Autodesk Inventor part; units mm, degrees
ref_plane "YZ Plane" through (0, 0, 0) normal (1, 0, 0) x (0, 1, 0)
ref_plane "XZ Plane" through (0, 0, 0) normal (0, 1, 0) x (-1, 0, 0)
ref_plane "XY Plane" through (0, 0, 0) normal (0, 0, 1) x (1, 0, 0)
sketch "Sketch2" plane through (0, 0, 0) normal (1, 0, 0) x (0, 1, 0)
  line L0 (0, 0) -> (2.5, 0)
  line L1 (2.5, 0) -> (2.5, -5.3)
  line L2 (2.5, -5.3) -> (2.15, -5.3)
  line L3 (2.15, -5.3) -> (2.15, -14.7)
  line L4 (2.15, -14.7) -> (2.5, -14.7)
  line L5 (2.5, -14.7) -> (2.5, -20)
  line L6 (2.5, -20) -> (0, -20)
  line L7 (0, -20) -> (0, 0)
  dimension "d1" = 2.5
  dimension "d2" = 5.3
  dimension "d3" = 0.35
  dimension "d4" = 9.4
  dimension "d5" = 0.35
  dimension "d6" = 5.3
  dimension "d7" = 2.5
revolve "Revolution1" add sketch "Sketch2" angle 360 about axis through (0, 0, -20) along (0, 0, 1)
fillet "Fillet4" radius 0.4 2 edges at (0, -2.5, -20) (0, -2.5, 0)
fillet "Fillet5" radius 0.35 2 edges at (0, -2.5, -14.7) (0, -2.5, -5.3)
equation "\"d5\" = d3"
equation "\"d6\" = d2"
equation "\"d7\" = d1"
properties part number "Fusible de 2A"
Verification items for the finished model (mm, model axes). Coordinates: 2 decimals unless noted, no trailing zeros. Order: outer loops, then holes, each group sorted by start corner. A loop starts at its lowest first (then second) coordinate and runs counter-clockwise, first axis right, second up. Notation, with made-up numbers: (51.5, 36.25) -> (64.5, 36.25) arc R9 ccw to (64.5, 42.25) -> close; hole circle Ø8 at (12.25, 2). An arc over 180 degrees is marked (long way). Answer as CSV lines item,"result". Start each with the question number.
1) Gauge pin test, flat end, axial feed: pin 1 Ø3 at (x, z) = (0.5, -12) entering from +Y. Record the tip position at first contact, or that the pin passes through.
2) Material ranges on L1, parallel to Z at x = 0.95, y = 2.1; L2, parallel to Y at x = 0.05, z = -10.75; L3, parallel to Y at x = -0.7, z = -3, recorded low to high. Write a range as [from, to].
3) Release check for a two-part mould opening along Z. For faces 1 (the face through (0, 0, -20)), 2 (the face through (-2.44, -0.54, -17.36)), 3 (the face through (0, 0, 0)), 4 (the face through (0.09, -2.15, -10.07)) record: released by +Z, released by -Z, zero draft, split by the parting line, or undercut.
4) Cross-section at D-D, the plane z = -7. Record the boundary of the cut face in (x, y), then the cut area to 3 significant figures.
5) Cross-section at C-C, the plane z = -18.5. Record the boundary of the cut face in (x, y), then the cut area to 3 significant figures.
Conclusion:
1,pin 1,"stops at y = 2.15"
2,L1,"z = [-19.94, -14.74], [-5.26, -0.06]"
2,L2,"y = [-2.15, 2.15]"
2,L3,"y = [-2.4, 2.4]"
3,face 1,"released by -Z"
3,face 2,"zero draft"
3,face 3,"released by +Z"
3,face 4,"undercut"
4,outline,"circle Ø4.3 at (0, 0)"
4,area,"14.5 mm²"
5,outline,"circle Ø5 at (0, 0)"
5,area,"19.6 mm²"
